Build history of the part. All positions in model axes, mm. A direction names the side the tool comes from. Coordinates: 2 decimals unless noted, no trailing zeros. Order: outer loops, then holes, each group sorted by start corner. A loop starts at its lowest first (then second) coordinate and runs counter-clockwise, first axis right, second up. Notation, with made-up numbers: (45.25, 50) -> (87.25, 50) arc R18 ccw to (87.25, 83) -> close; hole circle Ø10 at (36, -31). An arc over 180 degrees is marked (long way). Write each question's results on one line, items separated by ' | '.
Autodesk Fusion 360 part; units mm, degrees
sketch "Sketch1" plane through (0, 0, 0) normal (0, 0, 1) x (1, 0, 0)
  line L0 (-52.2, -60) -> (52.2, -60)
  line L1 (52.2, -60) -> (52.2, 60)
  line L2 (52.2, 60) -> (-52.2, 60)
  line L3 (-52.2, 60) -> (-52.2, -60)
  dimension "d1" = 104.4
  dimension "d2" = 120
  dimension "d3" = 60
  dimension "d4" = 52.2
extrude "Extrude1" add sketch "Sketch1" along normal blind 3
sketch "Sketch2" plane through (0, 0, 3) normal (0, 0, 1) x (-1, 0, 0)
  line L0 (52.2, -60) -> (52.2, 60)
  line L1 (52.2, 60) -> (-52.2, 60)
  line L2 (-52.2, 60) -> (-52.2, -60)
  line L3 (-52.2, -60) -> (52.2, -60)
  circle A0 centre (-48.2, -56) radius 1.5
  circle A1 centre (48.2, -56) radius 1.5
  circle A2 centre (48.2, 56) radius 1.5
  circle A3 centre (-48.2, 56) radius 1.5
  dimension "d7" = 3
  dimension "d8" = 3
  dimension "d9" = 3
  dimension "d10" = 3
  dimension "d11" = 4
  dimension "d12" = 4
  dimension "d13" = 4
  dimension "d14" = 4
  dimension "d15" = 4
  dimension "d16" = 4
  dimension "d17" = 4
  dimension "d18" = 4
hole "Hole1" at (-48.2, 56, 3) at (48.2, 56, 3) at (48.2, -56, 3) at (-48.2, -56, 3) direction (0, 0, -1) diameter 3 depth 3 tip angle 118
sketch "Sketch4" plane through (0, 0, 3) normal (0, 0, 1) x (-1, 0, 0)
  circle A0 centre (-48.2, 56) radius 1.5
  circle A1 centre (48.2, -56) radius 1.5
  circle A2 centre (-48.2, -56) radius 1.5
  circle A3 centre (48.2, 56) radius 1.5
  line L0 (52.2, -60) -> (52.2, 60)
  line L1 (52.2, 60) -> (-52.2, 60)
  line L2 (-52.2, 60) -> (-52.2, -60)
  line L3 (-52.2, -60) -> (52.2, -60)
  line L4 (40, -45) -> (35, -45)
  line L5 (35, -45) -> (35, 45)
  line L6 (35, 45) -> (40, 45)
  line L7 (40, 45) -> (40, -45)
  line L8 (10, -45) -> (10, 45)
  line L9 (10, 45) -> (15, 45)
  line L10 (15, 45) -> (15, -45)
  line L11 (15, -45) -> (10, -45)
  line L12 (-15, -45) -> (-15, 45)
  line L13 (-15, 45) -> (-10, 45)
  line L14 (-10, 45) -> (-10, -45)
  line L15 (-10, -45) -> (-15, -45)
  line L16 (-40, -45) -> (-40, 45)
  line L17 (-40, 45) -> (-35, 45)
  line L18 (-35, 45) -> (-35, -45)
  line L19 (-35, -45) -> (-40, -45)
  dimension "d39" = -75
  dimension "d40" = 0
  dimension "d41" = 5
  dimension "d42" = 90
  dimension "d43" = 40
  dimension "d44" = 45
extrude "Extrude2" cut sketch "Sketch4" against normal blind 3 contours L4 L5 L6 L7 | L8 L9 L10 L11 | L12 L13 L14 L15 | L16 L17 L18 L19
sketch "Sketch6" plane through (0, 0, 3) normal (0, 0, 1) x (-1, 0, 0)
  line L0 (10, 45) -> (15, 45)
  line L1 (15, 45) -> (15, -45)
  line L2 (15, -45) -> (10, -45)
  line L3 (10, -45) -> (10, 45)
  line L4 (-15, 45) -> (-10, 45)
  line L5 (-10, 45) -> (-10, -45)
  line L6 (-10, -45) -> (-15, -45)
  line L7 (-15, -45) -> (-15, 45)
  line L8 (35, -45) -> (35, 45)
  line L9 (35, 45) -> (40, 45)
  line L10 (40, 45) -> (40, -45)
  line L11 (40, -45) -> (35, -45)
  line L12 (-40, 45) -> (-35, 45)
  line L13 (-35, 45) -> (-35, -45)
  line L14 (-35, -45) -> (-40, -45)
  line L15 (-40, -45) -> (-40, 45)
  circle A0 centre (-48.2, 56) radius 1.5
  circle A1 centre (48.2, -56) radius 1.5
  circle A2 centre (-48.2, -56) radius 1.5
  circle A3 centre (48.2, 56) radius 1.5
  line L16 (52.2, -60) -> (52.2, 60)
  line L17 (52.2, 60) -> (-52.2, 60)
  line L18 (-52.2, 60) -> (-52.2, -60)
  line L19 (-52.2, -60) -> (52.2, -60)
  line L20 (-15, 25) -> (15, 25)
  line L21 (15, 25) -> (15, -25)
  line L22 (15, -25) -> (-15, -25)
  line L23 (-15, -25) -> (-15, 25)
  line L24 (-15, 25) -> (15, -25) construction
  line L25 (15, 25) -> (-15, -25) construction
  line L26 (40, -8) -> (35, -8)
  line L27 (35, -8) -> (35, 8)
  line L28 (35, 8) -> (40, 8)
  line L29 (40, 8) -> (40, -8)
  line L30 (-35, -8) -> (-40, -8)
  line L31 (-40, -8) -> (-40, 8)
  line L32 (-40, 8) -> (-35, 8)
  line L33 (-35, 8) -> (-35, -8)
  dimension "d49" = 50
  dimension "d56" = 8
  dimension "d57" = 16
  dimension "d58" = 8
  dimension "d59" = 16
extrude "Extrude3" add sketch "Sketch6" against normal blind 3 contours L1 L3 L20 L21 L22 | L5 L7 L20 L22 L23 | L8 L10 L26 L27 L28 L29 | L13 L15 L30 L31 L32 L33
sketch "Sketch5" plane through (0, 0, 3) normal (0, 0, 1) x (-1, 0, 0)
  line L0 (10, 45) -> (15, 45)
  line L1 (15, 45) -> (15, 25)
  line L2 (15, -45) -> (10, -45)
  line L3 (10, 25) -> (10, 45)
  line L4 (-15, 45) -> (-10, 45)
  line L5 (-10, -25) -> (-10, -45)
  line L6 (-10, -45) -> (-15, -45)
  line L7 (-15, -45) -> (-15, -25)
  line L8 (35, 8) -> (35, 45)
  line L9 (35, 45) -> (40, 45)
  line L10 (40, 45) -> (40, 8)
  line L11 (40, -45) -> (35, -45)
  line L12 (-40, 45) -> (-35, 45)
  line L13 (-35, 45) -> (-35, 8)
  line L14 (-35, -45) -> (-40, -45)
  line L15 (-40, 8) -> (-40, 45)
  circle A0 centre (-48.2, 56) radius 1.5
  circle A1 centre (48.2, -56) radius 1.5
  circle A2 centre (-48.2, -56) radius 1.5
  circle A3 centre (48.2, 56) radius 1.5
  line L16 (52.2, -60) -> (52.2, 60)
  line L17 (52.2, 60) -> (-52.2, 60)
  line L18 (-52.2, 60) -> (-52.2, -60)
  line L19 (-52.2, -60) -> (52.2, -60)
  circle A4 centre (0, 0) radius 11.25
  circle A5 centre (0, 0) radius 15
  line L20 (15, 25) -> (10, 25)
  line L21 (-15, -25) -> (-10, -25)
  line L22 (10, -25) -> (15, -25)
  line L23 (15, -25) -> (15, -45)
  line L24 (10, -45) -> (10, -25)
  line L25 (-10, 25) -> (-15, 25)
  line L26 (-15, 25) -> (-15, 45)
  line L27 (-10, 45) -> (-10, 25)
  line L28 (-35, 8) -> (-40, 8)
  line L29 (40, 8) -> (35, 8)
  line L30 (35, -8) -> (40, -8)
  line L31 (40, -8) -> (40, -45)
  line L32 (35, -45) -> (35, -8)
  line L33 (-40, -8) -> (-35, -8)
  line L34 (-35, -8) -> (-35, -45)
  line L35 (-40, -45) -> (-40, -8)
  dimension "d47" = 22.5
  dimension "d48" = 30
extrude "Extrude4" add sketch "Sketch5" along normal blind 30 contours A5
fillet "Fillet1" radius 6 1 edges at (13.9849, -5.4242, 3)
chamfer "Chamfer1" distance 0.5 angle 45 1 edges at (10.4887, -4.0682, 33)
sketch "Sketch7" plane through (0, 0, 0) normal (0, 1, 0) x (1, 0, 0)
  circle A0 centre (-0.0436, -26) radius 1.5
  dimension "d61" = 26
  dimension "d62" = 3
hole "Hole3" at (-0.0436, 0, 26) direction (0, -1, 0) diameter 3 depth 17 tip angle 118
thread "Thread1"
pattern_circular "C-Pattern1" count 3 over 360 about axis through (0, 0, 1.75) along (0, 0, 1) of "Hole3"
hole "Hole4" at (0, 0, 3) direction (0, 0, -1) diameter 16 depth 3 tip angle 118
sketch "Sketch8" plane through (0, 0, 0) normal (0, 0, -1) x (1, 0, 0)
  circle A0 centre (0, 0) radius 8
  line L0 (40, -8) -> (40, -45)
  line L1 (40, -45) -> (35, -45)
  line L2 (35, -45) -> (35, -8)
  line L3 (35, -8) -> (40, -8)
  line L4 (-10, -25) -> (-10, -45)
  line L5 (-10, -45) -> (-15, -45)
  line L6 (-15, -45) -> (-15, -25)
  line L7 (-15, -25) -> (-10, -25)
  line L8 (-35, -8) -> (-35, -45)
  line L9 (-35, -45) -> (-40, -45)
  line L10 (-40, -45) -> (-40, -8)
  line L11 (-40, -8) -> (-35, -8)
  line L12 (10, 25) -> (10, 45)
  line L13 (10, 45) -> (15, 45)
  line L14 (15, 45) -> (15, 25)
  line L15 (15, 25) -> (10, 25)
  line L16 (-10, 25) -> (-15, 25)
  line L17 (-15, 25) -> (-15, 45)
  line L18 (-15, 45) -> (-10, 45)
  line L19 (-10, 45) -> (-10, 25)
  line L20 (10, -25) -> (15, -25)
  line L21 (15, -25) -> (15, -45)
  line L22 (15, -45) -> (10, -45)
  line L23 (10, -45) -> (10, -25)
  line L24 (-35, 8) -> (-40, 8)
  line L25 (-40, 8) -> (-40, 45)
  line L26 (-40, 45) -> (-35, 45)
  line L27 (-35, 45) -> (-35, 8)
  line L28 (40, 8) -> (35, 8)
  line L29 (35, 8) -> (35, 45)
  line L30 (35, 45) -> (40, 45)
  line L31 (40, 45) -> (40, 8)
  circle A1 centre (48.2, 56) radius 1.5
  circle A2 centre (-48.2, -56) radius 1.5
  circle A3 centre (48.2, -56) radius 1.5
  circle A4 centre (-48.2, 56) radius 1.5
  line L32 (-52.2, 60) -> (-52.2, -60)
  line L33 (-52.2, -60) -> (52.2, -60)
  line L34 (52.2, -60) -> (52.2, 60)
  line L35 (52.2, 60) -> (-52.2, 60)
  line L36 (-21.595, 55.595) -> (21.595, 55.595)
  line L37 (21.595, 55.595) -> (21.595, 12.405)
  line L38 (21.595, 12.405) -> (-21.595, 12.405)
  line L39 (-21.595, 12.405) -> (-21.595, 55.595)
  line L40 (-25.4, -12.405) -> (25.4, -12.405)
  line L41 (25.4, -12.405) -> (25.4, -55.595)
  line L42 (25.4, -55.595) -> (-25.4, -55.595)
  line L43 (-25.4, -55.595) -> (-25.4, -12.405)
  line L44 (-19.055, 53.055) -> (19.055, 53.055)
  line L45 (19.055, 53.055) -> (19.055, 14.945)
  line L46 (19.055, 14.945) -> (-19.055, 14.945)
  line L47 (-19.055, 14.945) -> (-19.055, 53.055)
  line L48 (-22.86, -14.945) -> (22.86, -14.945)
  line L49 (22.86, -14.945) -> (22.86, -53.055)
  line L50 (22.86, -53.055) -> (-22.86, -53.055)
  line L51 (-22.86, -53.055) -> (-22.86, -14.945)
  dimension "d71" = 43.19
  dimension "d72" = 43.19
  dimension "d73" = 50.8
  dimension "d74" = 43.19
  dimension "d75" = 2.54
  dimension "d76" = 2.54
  dimension "d77" = 2.54
  dimension "d78" = 2.54
  dimension "d79" = 2.54
  dimension "d80" = 2.54
  dimension "d81" = 2.54
  dimension "d82" = 2.54
  dimension "d83" = 25.4
  dimension "d84" = 21.595
  dimension "d85" = 4.405
  dimension "d86" = 4.405
hole "Hole5" at (-19.055, -53.055, 0) at (19.055, -53.055, 0) at (19.055, -14.945, 0) at (-19.055, -14.945, 0) at (-22.86, 14.945, 0) at (-22.86, 53.055, 0) at (22.86, 53.055, 0) at (22.86, 14.945, 0) direction (0, 0, 1) diameter 3 depth 3 tip angle 118
Item 1: Slice it at B-B, the plane x = 22.86. List the corners of the cut face in (y, z) (3 decimals).
Answer:
outline: (-60, 0) -> (13.445, 0) -> (13.445, 3) -> (-60, 3) -> close; (16.445, 0) -> (51.555, 0) -> (51.555, 3) -> (16.445, 3) -> close; (54.555, 0) -> (60, 0) -> (60, 3) -> (54.555, 3) -> close
Item 2: Slice it at D-D, the plane y = 0. List the corners of the cut face in (x, z).
Answer:
outline: (-52.2, 0) -> (-8, 0) -> (-8, 3) -> (-11.25, 3) -> (-11.25, 32.5) -> (-11.75, 33) -> (-15, 33) -> (-15, 9) arc R6 cw to (-21, 3) -> (-52.2, 3) -> close; (8, 0) -> (52.2, 0) -> (52.2, 3) -> (21, 3) arc R6 cw to (15, 9) -> (15, 33) -> (11.75, 33) -> (11.25, 32.5) -> (11.25, 3) -> (8, 3) -> close
Item 3: Slice it at C-C, the plane y = -56. List the corners of the cut face in (x, z).
Answer:
outline: (-52.2, 0) -> (-49.7, 0) -> (-49.7, 3) -> (-52.2, 3) -> close; (-46.7, 0) -> (46.7, 0) -> (46.7, 3) -> (-46.7, 3) -> close; (49.7, 0) -> (52.2, 0) -> (52.2, 3) -> (49.7, 3) -> close
Item 4: Drill centre lines: line 1 (Y direction, x = -22.86, z = 1.15) (3 decimals); line 2 (Y direction, x = -48, z = 1); line 3 (X direction, y = -56, z = 2). Where is each one in solid material? Low to high. Write a range as from..to.
Answer:
line 1: y = -60..13.445, 16.445..51.555, 54.555..60 | line 2: y = -60..-57.49, -54.51..54.51, 57.49..60 | line 3: x = -52.2..-49.7, -46.7..46.7, 49.7..52.2
Item 5: Pin check, flat tips, straight feed: pin 1 (3 mm diameter, centred on y = 5.5, z = 27.5, fed in from +X); pin 2 (12 mm diameter, centred on x = -15.5, z = 14, fed in from -Y); pin 3 (12 mm diameter, centred on y = 14, z = 9.5, fed in from -X). Stop position of each tip, or through.
Answer:
pin 1: stops at x = 14.46 | pin 2: stops at y = -11.61 | pin 3: stops at x = -13.35
Item 6: Pull direction X, two halves, no side cores. Call faces 1 (the flat face through (22, 1, 3)), 2 (the flat face through (37, 45, 2)), 3 (the flat face through (52.2, -1, 1)): released by +X, released by -X, zero draft, split by the parting line, or undercut.
Answer:
face 1: zero draft | face 2: undercut | face 3: released by +X
Item 7: Slice it at A-A, the plane y = -42.5. List the corners of the cut face in (x, z).
Answer:
outline: (-52.2, 0) -> (-40, 0) -> (-40, 3) -> (-52.2, 3) -> close; (-35, 0) -> (-15, 0) -> (-15, 3) -> (-35, 3) -> close; (-10, 0) -> (10, 0) -> (10, 3) -> (-10, 3) -> close; (15, 0) -> (35, 0) -> (35, 3) -> (15, 3) -> close; (40, 0) -> (52.2, 0) -> (52.2, 3) -> (40, 3) -> close
Item 8: Tool access for faces 4 (the flat face through (35, 26, 2)), 5 (the cylindrical face through (-11.1, 6.98, 27.43)), 6 (the cylindrical face through (-5.19, -9.98, 17.54)): list every direction of +Z, -Z, +X, -X, +Y, -Y with a clear straight run to the whole face (end or side of a thin tool).
Answer:
face 4: +Z, -Z | face 5: none | face 6: +Z
